Geometry check sheet. Reference: the model listing, model coordinates, mm. A direction names the side the tool comes from. Coordinates: 2 decimals unless noted, no trailing zeros. Loops run counter-clockwise (first coordinate to the right, second up) from the corner with the lowest first, then second, coordinate; pieces in that order, holes last.
from build123d import *

# Parameters (mm, degrees)
PAD029_DEPTH                  = 20
PAD029_DEPTH_BACK             = 22
POCKET050_DEPTH               = 130.2017462661
POCKET050_MIRRORED022_2_DEPTH = 130.2017462661
PAD052_DEPTH                  = 25
SKETCH105_R                   = 3.9
POCKET053_DEPTH               = 0.001
POCKET053_DEPTH_BACK          = 30.001


with BuildPart() as part:
    # Sketch053 → Pad029 (new body, two sides)
    with BuildSketch(Plane.YZ) as pad029_sk:
        with BuildLine():
            Line((-7, 5), (-7, 10))
            Line((-7, 10), (4, 10))
            ThreePointArc((4, 10), (8.2426406871, 11.7573593129), (10, 16))
            Line((10, 16), (10, 30))
            Line((10, 30), (15, 30))
            Line((15, 30), (15, 5))
            Line((15, 5), (-7, 5))
        make_face()
    extrude(amount=-PAD029_DEPTH)
    extrude(pad029_sk.sketch, amount=PAD029_DEPTH_BACK)

    # Sketch100 → Pocket050 (cut, through all)
    with BuildSketch(Plane(origin=(0, 0, 7), x_dir=(-1, 0, 0), z_dir=(0, 0, -1))):
        with BuildLine():
            ThreePointArc((0, 3.95), (-2.7930717857, 2.7930717857), (-3.95, 0))
            Line((-3.95, 0), (18.2, 0))
            ThreePointArc((18.2, 0), (17.6374362231, 1.4692864307), (16.2374521678, 2.1871480215))
            Line((0, 3.95), (16.2374521678, 2.1871480215))
        make_face()
    pocket050 = extrude(amount=-POCKET050_DEPTH, mode=Mode.SUBTRACT)

    # Sketch100 Mirrored022 2 → Pocket050 Mirrored022 2 (cut, through all)
    with BuildSketch(Plane.XY.offset(7)):
        with BuildLine():
            ThreePointArc((0, 3.95), (-2.7930717857, 2.7930717857), (-3.95, 0))
            Line((-3.95, 0), (18.2, 0))
            ThreePointArc((18.2, 0), (17.6374362231, 1.4692864307), (16.2374521678, 2.1871480215))
            Line((0, 3.95), (16.2374521678, 2.1871480215))
        make_face()
    pocket050_mirrored022_2 = extrude(amount=POCKET050_MIRRORED022_2_DEPTH, mode=Mode.SUBTRACT)

    # Mirrored023: Pocket050, Pocket050 Mirrored022 2 across Sketch100 H_Axis
    add(pocket050.mirror(Plane(origin=(0, 0, 7), x_dir=(0, 0, -1), z_dir=(0, 1, 0))), mode=Mode.SUBTRACT)
    add(pocket050_mirrored022_2.mirror(Plane(origin=(0, 0, 7), x_dir=(0, 0, -1), z_dir=(0, 1, 0))), mode=Mode.SUBTRACT)

    # Sketch101 (on Face2 of MultiTransform004) → Pad052 (join)
    with BuildSketch(Plane.YX.offset(-5)):
        Polygon((15, 22), (25, 22), (25, 15.3205080757), (15, 18), align=None)
    extrude(amount=-PAD052_DEPTH)

    # Sketch105 → Pocket053 (cut, two sides)
    with BuildSketch(Plane.XY) as pocket053_sk:
        Circle(SKETCH105_R)
    extrude(amount=-POCKET053_DEPTH, mode=Mode.SUBTRACT)
    extrude(pocket053_sk.sketch, amount=POCKET053_DEPTH_BACK, mode=Mode.SUBTRACT)


solid = part.part
(1) Gauge pin test, flat ends, axial feed: pin 1 Ø2 at (x, z) = (-6, 22) entering from +Y; pin 2 Ø9 at (x, y) = (11, -3) entering from +Z; pin 3 Ø4.5 at (x, y) = (0, 0) entering from -Z; pin 4 Ø7 at (x, z) = (0.5, 26.5) entering from -Y. Record the tip position at first contact, or that the pin passes through.
Findings:
pin 1: stops at y = 15
pin 2: stops at z = 10
pin 3: passes through
pin 4: stops at y = 10
(2) Scan lines: L1, parallel to Y at x = 0, z = 6.5; L2, parallel to X at y = 0, z = 6.35; L3, parallel to Y at x = -18, z = 25.25. Record each from-to range of solid material in increasing order.
Findings:
L1: y = -7 to -3.9, 3.9 to 15
L2: x = -20 to -3.9, 3.9 to 22
L3: y = 10 to 15
(3) Access from +Z, -Z, +X, -X, +Y, -Y to the whole of each face (thin tool, end or side, straight path). Record for faces 4 (the flat face through (1, 6, 5)), 5 (the flat face through (1, 10, 23)), 6 (the flat face through (16.64, 20.07, 17.32)), 7 (the flat face through (6, 14, 30)), 8 (the flat face through (-8.435, 3.034, 8.479)).
Findings:
face 4: -Z, +X, -X, +Y, -Y
face 5: +Z, +X, -X, -Y
face 6: +Z, -Z, -X
face 7: +Z, +X, -X, +Y, -Y
face 8: +Z
(4) Sectioned sample at A-A on z = 8. Record the cut outline in (x, y).
Findings:
outline: (-20, -7) - (22, -7) - (22, 25) - (15.32, 25) - (18, 15) - (-20, 15) - close; hole (-16.24, -2.19) - (-0.85, -3.86) arc R3.95 ccw to (0.85, -3.86) - (16.24, -2.19) arc R2.2 ccw to (16.24, 2.19) - (0.85, 3.86) arc R3.95 ccw to (-0.85, 3.86) - (-16.24, 2.19) arc R2.2 ccw to start
(5) Sectioned sample at D-D on x = -10. Record the cut outline in (y, z), and give its area (3 significant figures).
Findings:
outline: (-7, 5) - (15, 5) - (15, 30) - (10, 30) - (10, 16) arc R6 cw to (4, 10) - (2.86, 10) - (2.86, 7) - (-2.86, 7) - (-2.86, 10) - (-7, 10) - close
area: 201 mm2
(6) Sectioned sample at B-B on x = 1.5. Record the cut outline in (y, z).
Findings:
outline: (-7, 5) - (-3.6, 5) - (-3.6, 7) - (-3.79, 7) - (-3.79, 10) - (-7, 10) - close; (3.6, 5) - (15, 5) - (15, 30) - (10, 30) - (10, 16) arc R6 cw to (4, 10) - (3.79, 10) - (3.79, 7) - (3.6, 7) - close
(7) Draft check along X on faces 1 (the flat face through (19, 25, 17)), 2 (the flat face through (22, 12, 15)), 3 (the cylindrical face through (-2.87, 2.64, 5.99)). Enter one of: +X half, -X half, draft (parallel to the pull), parting line (faces both ways), or undercut.
Findings:
face 1: draft
face 2: +X half
face 3: undercut
(8) Sectioned sample at C-C on y = -0.5. Record the cut outline in (x, z), and give its area (3 significant figures).
Findings:
outline: (-20, 5) - (-3.87, 5) - (-3.87, 7) - (-18.14, 7) - (-18.14, 10) - (-20, 10) - close; (3.87, 5) - (22, 5) - (22, 10) - (18.14, 10) - (18.14, 7) - (3.87, 7) - close
area: 85.7 mm2
